Can you work these out from the model? Positions are in its coordinate system, mm. Coordinates: 2 decimals unless noted, no trailing zeros. Order: outer loops, then holes, each group sorted by start corner. A loop starts at its lowest first (then second) coordinate and runs counter-clockwise, first axis right, second up. Notation, with made-up numbers: M -21,61.5 L -5,61.5 A14 cw -5,66.5 Z; hole C 86.5,6.25 d7. An arc over 180 degrees is marked long. Answer as CSV lines item,"result". Start each with the question number.
1. If we section it at A-A (x = 269.5): List the corners of the cut face in (y, z) for me, plus the area to 3 significant figures.
2. If we section it at B-B (z = 13.25): Give the number of separate pieces and of enclosed holes in the cut face, plus the area to 3 significant figures.
3. Will this pin go through, and if not, where does the flat tip stop? pin 1 (5.5 mm diameter, centred on x = 200.5, z = 8.5, fed in from +Y).
4. If we section it at C-C (x = 175.5): List the corners of the cut face in (y, z) for me.
5. I need wall thicknesses on line 1 along Y through (x, z) = (108.5, 8.75); line 2 along Y through (x, z) = (383.5, 12.5). Which ranges of each line are inside material? Lowest first, please. Write a range as from..to.
Autodesk Inventor part; units mm, degrees
ref_plane "YZ Plane" through (0, 0, 0) normal (1, 0, 0) x (0, 1, 0)
ref_plane "XZ Plane" through (0, 0, 0) normal (0, 1, 0) x (-1, 0, 0)
ref_plane "XY Plane" through (0, 0, 0) normal (0, 0, 1) x (1, 0, 0)
sketch "Sketch1" plane through (0, 0, 0) normal (0, 0, 1) x (1, 0, 0)
  line L0 (0, 0) -> (400, 0)
  line L1 (400, 0) -> (400, 1000)
  line L2 (0, 1000) -> (0, 0)
  line L3 (80, 1002.5) -> (80, 1018)
  line L4 (160, 1002.5) -> (160, 1018)
  line L5 (240, 1002.5) -> (240, 1018)
  line L6 (320, 1002.5) -> (320, 1018)
  line L7 (80, 1018) -> (160, 1018)
  line L8 (240, 1018) -> (320, 1018)
  line L9 (400, 1000) -> (322.5, 1000)
  line L10 (237.5, 1000) -> (162.5, 1000)
  arc A0 (77.5, 1000) -> (80, 1002.5) centre (80, 1000) ccw
  arc A1 (160, 1002.5) -> (162.5, 1000) centre (160, 1000) ccw
  arc A2 (237.5, 1000) -> (240, 1002.5) centre (240, 1000) ccw
  arc A3 (320, 1002.5) -> (322.5, 1000) centre (320, 1000) ccw
  line L11 (0, 1000) -> (77.5, 1000)
  line L12 (80, 697.5) -> (80, 684.5)
  line L13 (160, 697.5) -> (160, 684.5)
  line L14 (240, 697.5) -> (240, 684.5)
  line L15 (320, 697.5) -> (320, 684.5)
  line L16 (82.5, 682) -> (157.5, 682)
  line L17 (242.5, 682) -> (317.5, 682)
  line L18 (82.5, 700) -> (157.5, 700)
  line L19 (242.5, 700) -> (317.5, 700)
  line L20 (80, 379.5) -> (80, 366.5)
  line L21 (80, 61.5003) -> (80, 48.5)
  line L22 (160, 379.5003) -> (160, 366.5)
  line L23 (160, 61.5003) -> (160, 48.5)
  line L24 (240, 379.5) -> (240, 366.5)
  line L25 (240, 61.5) -> (240, 48.5)
  line L26 (320, 379.5) -> (320, 366.4997)
  line L27 (320, 61.5003) -> (320, 48.5)
  line L28 (82.5, 382) -> (157.4609, 382)
  line L29 (82.5, 364) -> (157.5, 364)
  line L30 (242.5, 364) -> (317.4609, 364)
  line L31 (82.5, 64) -> (157.4609, 64)
  line L32 (242.5, 64) -> (317.4609, 64)
  line L33 (82.5, 46) -> (157.5, 46)
  line L34 (242.5, 46) -> (317.5, 46)
  arc A4 (82.5, 700) -> (80, 697.5) centre (80, 700) ccw
  arc A5 (160, 697.5) -> (157.5, 700) centre (160, 700) ccw
  arc A6 (157.5, 682) -> (160, 684.5) centre (160, 682) ccw
  arc A7 (80, 684.5) -> (82.5, 682) centre (80, 682) ccw
  arc A8 (242.5, 700) -> (240, 697.5) centre (240, 700) ccw
  arc A9 (240, 684.5) -> (242.5, 682) centre (240, 682) ccw
  arc A10 (320, 697.5) -> (317.5, 700) centre (320, 700) ccw
  arc A11 (317.5, 682) -> (320, 684.5) centre (320, 682) ccw
  arc A12 (320, 379.5) -> (317.5, 382) centre (320, 382) ccw
  arc A13 (317.4609, 364) -> (320, 366.4997) centre (319.9609, 364) ccw
  arc A14 (242.5, 382) -> (240, 379.5) centre (240, 382) ccw
  arc A15 (240, 366.5) -> (242.5, 364) centre (240, 364) ccw
  arc A16 (157.5, 364) -> (160, 366.5) centre (160, 364) ccw
  arc A17 (160, 379.5003) -> (157.4609, 382) centre (159.9609, 382) ccw
  arc A18 (82.5, 382) -> (80, 379.5) centre (80, 382) ccw
  arc A19 (80, 366.5) -> (82.5, 364) centre (80, 364) ccw
  arc A20 (82.5, 64) -> (80, 61.5003) centre (80, 64.0003) ccw
  arc A21 (160, 61.5003) -> (157.4609, 64) centre (159.9609, 64) ccw
  arc A22 (157.5, 46) -> (160, 48.5) centre (160, 46) ccw
  arc A23 (80, 48.5) -> (82.5, 46) centre (80, 46) ccw
  arc A24 (242.5, 64) -> (240, 61.5) centre (240, 64) ccw
  arc A25 (320, 61.5003) -> (317.4609, 64) centre (319.9609, 64) ccw
  arc A26 (317.5, 46) -> (320, 48.5) centre (320, 46) ccw
  arc A27 (240, 48.5) -> (242.5, 46) centre (240, 46) ccw
  line L35 (242.5, 382) -> (317.5, 382)
  dimension "d1" = 1000
  dimension "d4" = 80
  dimension "d5" = 80
  dimension "d6" = 80
  dimension "d7" = 400
  dimension "d9" = 5
  dimension "d10" = 5
  dimension "d11" = 5
  dimension "d12" = 5
  dimension "d19" = 80
  dimension "d20" = 80
  dimension "d21" = 80
  dimension "d22" = 80
  dimension "d23" = 18
  dimension "d24" = 18
  dimension "d31" = 80
  dimension "d33" = 80
  dimension "d34" = 80
  dimension "d38" = 18
  dimension "d41" = 18
  dimension "d42" = 18
  dimension "d43" = 80
  dimension "d44" = 80
  dimension "d45" = 80
  dimension "d46" = 80
  dimension "d47" = 5
  dimension "d48" = 5
  dimension "d49" = 5
  dimension "d50" = 5
  dimension "d51" = 5
  dimension "d52" = 5
  dimension "d53" = 5
  dimension "d54" = 5
  dimension "d55" = 5
  dimension "d56" = 5
  dimension "d57" = 5
  dimension "d58" = 5
  dimension "d59" = 5
  dimension "d60" = 5
  dimension "d61" = 5
  dimension "d62" = 5
  dimension "d63" = 5
  dimension "d64" = 5
  dimension "d65" = 5
  dimension "d66" = 5
  dimension "d67" = 5
  dimension "d68" = 5
  dimension "d69" = 5
  dimension "d70" = 5
  dimension "d71" = 80
  dimension "d72" = 18
extrude "Extrusion1" add sketch "Sketch1" along normal blind 18
properties part number "tapa laterales"
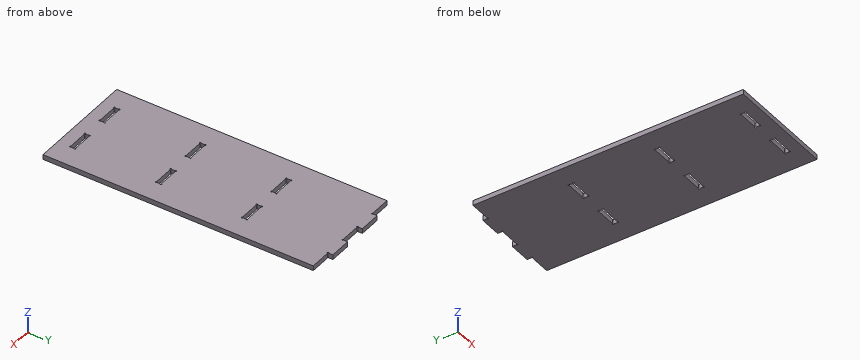
Solved:
1,outline,"M 0,0 L 46,0 L 46,18 L 0,18 Z; M 64,0 L 364,0 L 364,18 L 64,18 Z; M 382,0 L 682,0 L 682,18 L 382,18 Z; M 700,0 L 1018,0 L 1018,18 L 700,18 Z"
1,area,"17,400 mm²"
2,separate pieces,"1"
2,enclosed holes,"6"
2,area,"394,000 mm²"
3,pin 1,"y = 1000"
4,outline,"M 0,0 L 1000,0 L 1000,18 L 0,18 Z"
5,line 1,"0..46, 64..364, 382..682, 700..1018"
5,line 2,"0..1000"
